The listing builds one solid part. Answer for the finished solid, in the listing's coordinates (mm). A direction names the side the tool comes from. Coordinates: 2 decimals unless noted, no trailing zeros. Write each loop counter-clockwise with the first axis right and the second up, starting at its lowest first coordinate (ties: lowest second). Pieces come first, ordered by that corner, then holes.
from build123d import *

# Parameters (mm, degrees)
SKETCH1_W           = 3
SKETCH1_H           = 12
BOSS_EXTRUDE1_DEPTH = 40
CUT_EXTRUDE1_DEPTH  = 3
SKETCH3_R           = 0.5
CUT_EXTRUDE2_DEPTH  = 5
SKETCH4_W           = 12
SKETCH4_H           = 1.5
BOSS_EXTRUDE2_DEPTH = 5
SKETCH5_R           = 0.75
CUT_EXTRUDE3_DEPTH  = 5


with BuildPart() as part:
    # Sketch1 → Boss-Extrude1 (new body)
    with BuildSketch(Plane(origin=(0, 0, 0), x_dir=(1, 0, 0), z_dir=(0, 1, 0))):
        Rectangle(SKETCH1_W, SKETCH1_H)
    extrude(amount=BOSS_EXTRUDE1_DEPTH)

    # Sketch2 → Cut-Extrude1 (cut)
    with BuildSketch(Plane(origin=(1.5, 0, 0), x_dir=(0, 0, -1), z_dir=(1, 0, 0))):
        with BuildLine():
            Line((-2.5, 40), (-2.5, 37.5))
            ThreePointArc((-2.5, 37.5), (0, 35), (2.5, 37.5))
            Line((2.5, 37.5), (2.5, 40))
            Line((2.5, 40), (-2.5, 40))
        make_face()
    extrude(amount=-CUT_EXTRUDE1_DEPTH, mode=Mode.SUBTRACT)

    # Sketch3 → Cut-Extrude2 (cut)
    with BuildSketch(Plane(origin=(0, 40, 0), x_dir=(1, 0, 0), z_dir=(0, 1, 0))):
        with Locations((0, -4.25)):
            Circle(SKETCH3_R)
        with Locations((0, 4.25)):
            Circle(SKETCH3_R)
    extrude(amount=-CUT_EXTRUDE2_DEPTH, mode=Mode.SUBTRACT)

    # Sketch4 → Boss-Extrude2 (add)
    with BuildSketch(Plane(origin=(1.5, 0, 0), x_dir=(0, 0, -1), z_dir=(1, 0, 0))):
        with Locations((0, 0.75)):
            Rectangle(SKETCH4_W, SKETCH4_H)
    extrude(amount=BOSS_EXTRUDE2_DEPTH)

    # Sketch5 → Cut-Extrude3 (cut)
    with BuildSketch(Plane(origin=(0, 1.5, 0), x_dir=(1, 0, 0), z_dir=(0, 1, 0))):
        with Locations((4, 3)):
            Circle(SKETCH5_R)
        with Locations((4, -3)):
            Circle(SKETCH5_R)
    extrude(amount=-CUT_EXTRUDE3_DEPTH, mode=Mode.SUBTRACT)


solid = part.part
1. Section A-A on x = 4 is taken. Give the vertices of the cut face in (y, z), then the cut area to 3 significant figures.
Results found:
outline: (0, -6) - (1.5, -6) - (1.5, -3.75) - (0, -3.75) - close; (0, -2.25) - (1.5, -2.25) - (1.5, 2.25) - (0, 2.25) - close; (0, 3.75) - (1.5, 3.75) - (1.5, 6) - (0, 6) - close
area: 13.5 mm2
2. Flat-ended cylindrical pins translate along their axes: P1, Ø4, axis at x = 5, z = -2.5, coming from the +Y side; P2, Ø1.4, axis at x = 4, z = -3, coming from the -Y side; P3, Ø2, axis at y = 35.5, z = 0.5, coming from the +X side. Find the tip coordinate at first contact, or state that the pin passes through.
Results found:
P1: stops at y = 1.5
P2: passes through
P3: stops at x = 1.5
3. Section B-B on z = -4.25 is taken. Give the vertices of the cut face in (x, y), then the cut area to 4 significant figures.
Results found:
outline: (-1.5, 0) - (6.5, 0) - (6.5, 1.5) - (1.5, 1.5) - (1.5, 40) - (0.5, 40) - (0.5, 35) - (-0.5, 35) - (-0.5, 40) - (-1.5, 40) - close
area: 122.5 mm2
4. Section D-D on x = 2.5 is taken. Give the vertices of the cut face in (y, z).
Results found:
outline: (0, -6) - (1.5, -6) - (1.5, 6) - (0, 6) - close
5. Section C-C on y = 31.5 is taken. Give the vertices of the cut face in (x, z).
Results found:
outline: (-1.5, -6) - (1.5, -6) - (1.5, 6) - (-1.5, 6) - close
6. Find the intervals of material crossed by L1, parallel to Z at x = 4, y = 0.7; L2, parallel to Z at x = 0, y = 37.9; L3, parallel to X at y = 0.45, z = 3, in increasing order.
Results found:
L1: z = -6 to -3.75, -2.25 to 2.25, 3.75 to 6
L2: z = -6 to -4.75, -3.75 to -2.5, 2.5 to 3.75, 4.75 to 6
L3: x = -1.5 to 3.25, 4.75 to 6.5
7. A tool of negligible diameter and unlimited length cuts with its end or side. For faces 5 (the flat face through (0, 18, -6)), 6 (the flat face through (0, 35, -4)), 7 (the flat face through (0, 39, -2.5)), 8 (the flat face through (1.5, 20, 0)), from which of +Z, -Z, +X, -X, +Y, -Y can it reach the whole face along a straight path? Write none if from no direction.
Results found:
face 5: -Z, +X, -X, +Y, -Y
face 6: +Y
face 7: +X, -X, +Y
face 8: +Z, -Z, +X, +Y
8. For a pull along X with two mould halves and no side action, classify faces 1 (the flat face through (-1.5, 20, 0)), 2 (the cylindrical face through (3.405, 0.76, 3.456)), 3 (the cylindrical face through (3.405, 0.76, -2.544)), 4 (the flat face through (0, 39, 2.5)) as pulls with the +X half, pulls with the -X half, needs draft (parallel to the pull), parting line crosses it, or undercut.
Results found:
face 1: pulls with the -X half
face 2: undercut
face 3: undercut
face 4: needs draft
